Can you work these out from the drawing? Everything is in mm from the part's minimum corner. Give positions to 0.01 mm unless a question says otherwise; leave off trailing zeros. Loops run counter-clockwise (first coordinate to the right, second up) from the corner with the lowest first, then second, coordinate; pieces in that order, holes last.
Q1. If we section it at D-D (x = 62.5): Please give me the cut outline in (y, z).
Q2. If we section it at A-A (x = 45): Please give me the cut outline in (y, z).
Q3. Will these pins go through, and if not, where does the flat tip stop? P1, Ø2, axis at x = 39.5, y = 56.5, coming from the -Z side; P2, Ø1, axis at y = 12.5, z = 1.5, coming from the -X side (3 decimals); P3, Ø1.5, axis at y = 10.5, z = 2, coming from the -X side.
Q4. If we section it at B-B (z = 1.2): Please give me the cut outline in (x, y), plus the area to 3 significant figures.
Q5. I need wall thicknesses on line 1 (Y direction, x = 45, z = 2.2); line 2 (Y direction, x = 44, z = 1.45); line 3 (X direction, y = 59.5, z = 0.3). Which ranges of each line are inside material? Lowest first, please.
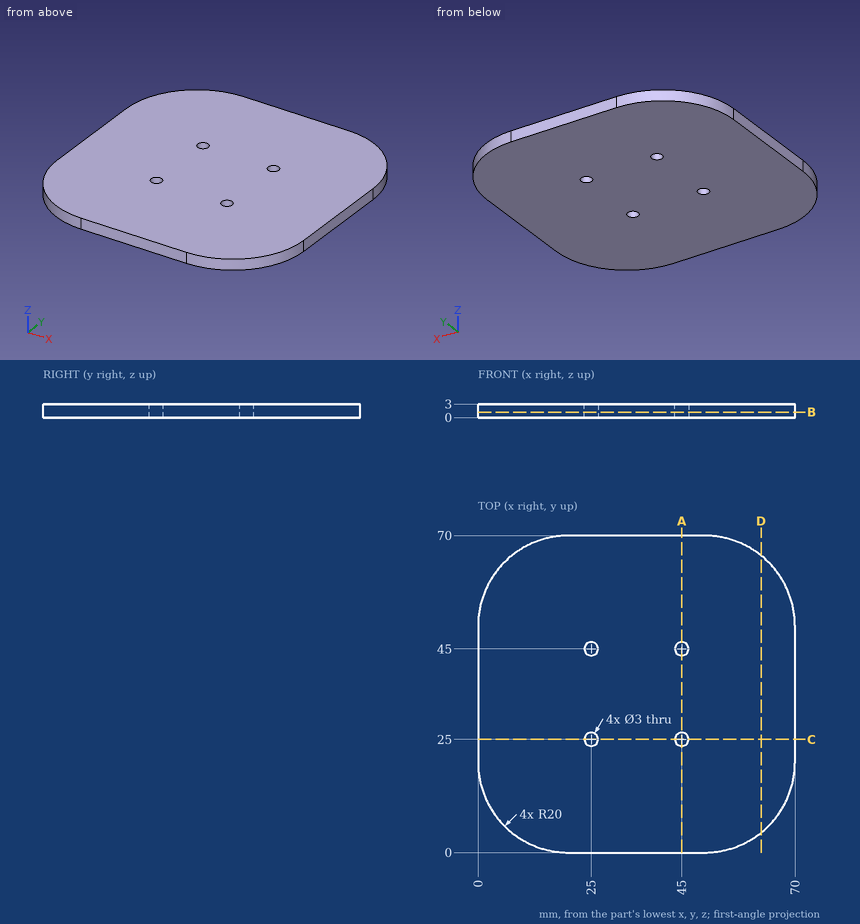
Check sheet entries:
1. outline: (4.39, 0) - (65.61, 0) - (65.61, 3) - (4.39, 3) - close
2. outline: (0, 0) - (23.5, 0) - (23.5, 3) - (0, 3) - close; (26.5, 0) - (43.5, 0) - (43.5, 3) - (26.5, 3) - close; (46.5, 0) - (70, 0) - (70, 3) - (46.5, 3) - close
3. P1: stops at z = 0
3. P2: stops at x = 1.265
3. P3: stops at x = 2.02
4. outline: (0, 20) arc R20 ccw to (20, 0) - (50, 0) arc R20 ccw to (70, 20) - (70, 50) arc R20 ccw to (50, 70) - (20, 70) arc R20 ccw to (0, 50) - close; hole circle Ø3 at (25, 25); hole circle Ø3 at (25, 45); hole circle Ø3 at (45, 25); hole circle Ø3 at (45, 45)
4. area: 4,530 mm2
5. line 1: y = 0 to 23.5, 26.5 to 43.5, 46.5 to 70
5. line 2: y = 0 to 23.88, 26.12 to 43.88, 46.12 to 70
5. line 3: x = 2.4 to 67.6
